Check sheet for the modelled part. Datum: model origin and axes. Units: mm. A direction names the side the tool comes from. Round coordinates to 2 decimals unless told otherwise and drop trailing zeros. Write each loop counter-clockwise with the first axis right and the second up, starting at its lowest first coordinate (ties: lowest second). Pieces come first, ordered by that corner, then holes. Notation, with made-up numbers: (-28.5, 34.5) -> (23.5, 34.5) arc R23 cw to (23.5, 48.5) -> close; hole circle Ø7 at (48, -26). An arc over 180 degrees is marked (long way). One line per item, written item: value.
Autodesk Inventor part; units mm, degrees
ref_plane "YZ Plane" through (0, 0, 0) normal (1, 0, 0) x (0, 1, 0)
ref_plane "XZ Plane" through (0, 0, 0) normal (0, 1, 0) x (-1, 0, 0)
ref_plane "XY Plane" through (0, 0, 0) normal (0, 0, 1) x (1, 0, 0)
sketch "スケッチ1" plane through (0, 0, 0) normal (0, 0, 1) x (1, 0, 0)
  circle A0 centre (0, 0) radius 1.5
  dimension "d0" = 3
extrude "押し出し1" add sketch "スケッチ1" along normal blind 20
sketch "スケッチ2" plane through (0, 0, 0) normal (0, 0, -1) x (-1, 0, 0)
  circle A0 centre (0, 0) radius 3
  dimension "d3" = 6
extrude "押し出し2" add sketch "スケッチ2" against normal blind 2
thread "ねじ1"
chamfer "面取り1" distance 1.5 angle 45 1 edges at (3, 0, 2)
properties part number "ネジ皿m3,20" material "鋼、高強度、低合金"
Item 1: Sectioned sample at C-C (z = 3.25). Enter the section's corners in (x, y), then the cut area to 3 significant figures.
Result set:
outline: circle Ø3 at (0, 0)
area: 7.07 mm^2
Item 2: Depth check by flat-ended pin: pin 1 (2 mm diameter, centred on x = -1.5, z = 9.5, fed in from -Y); pin 2 (2 mm diameter, centred on x = -2, z = 5.5, fed in from +Y); pin 3 (2 mm diameter, centred on x = 0.5, y = -2.5, fed in from -Z); pin 4 (1 mm diameter, centred on x = -1, z = 15.5, fed in from +Y). Enter the tip coordinate at first touch or a pass-through.
Result set:
pin 1: y = -1.41
pin 2: y = 1.12
pin 3: z = 0
pin 4: y = 1.41
Item 3: Material ranges on line 1 along Y through (x, z) = (0, 17.25); line 2 along Y through (x, z) = (-0.45, 9.25); line 3 along Z through (x, y) = (-1.5, 0.9), recorded low to high.
Result set:
line 1: -1.5 to 1.5
line 2: -1.43 to 1.43
line 3: 0 to 1.75
Item 4: Tool access check on faces 1 (the flat face through (0, 0, 0)), 2 (the cylindrical face through (-1.5, -0.07, 10.87)). Record the directions out of +Z, -Z, +X, -X, +Y, -Y that give a thin tool (end or side, any length) a straight path to the whole face; none if there is none.
Result set:
face 1: -Z, +X, -X, +Y, -Y
face 2: +Z
